```python
from build123d import *

# Parameters (mm, degrees)
SKETCH1_W           = 202.8
SKETCH1_H           = 130.8
SKETCH1_W_2         = 198
SKETCH1_H_2         = 126
BOSS_EXTRUDE1_DEPTH = 102
SKETCH3_W           = 198
SKETCH3_H           = 126
BOSS_EXTRUDE3_DEPTH = 2.4
FILLET1_R           = 5
FILLET4_R           = 10
FILLET2_R           = 6
FILLET3_R           = 0.4
CUT_EXTRUDE1_DEPTH  = 30


with BuildPart() as part:
    # Sketch1 → Boss-Extrude1 (new body)
    with BuildSketch(Plane(origin=(0, 0, 0), x_dir=(1, 0, 0), z_dir=(0, 1, 0))):
        with Locations((99, -63)):
            Rectangle(SKETCH1_W, SKETCH1_H)
        with Locations((99, -63)):
            Rectangle(SKETCH1_W_2, SKETCH1_H_2, mode=Mode.SUBTRACT)
    extrude(amount=BOSS_EXTRUDE1_DEPTH)

    # Sketch3 → Boss-Extrude3 (add)
    with BuildSketch(Plane(origin=(0, 0, 0), x_dir=(-1, 0, 0), z_dir=(0, -1, 0))):
        with Locations((-99, -63)):
            Rectangle(SKETCH3_W, SKETCH3_H)
    extrude(amount=-BOSS_EXTRUDE3_DEPTH)

    # Fillet1
    fillet1_edges = [part.edges().sort_by_distance(p)[0] for p in [
        (0, 2.4, 63),
        (99, 2.4, 126),
        (198, 2.4, 63),
        (99, 2.4, 0),
    ]]
    fillet(fillet1_edges, radius=FILLET1_R)

    # Fillet4
    # the kernel refuses this fillet: 10 mm, written as the material it adds along each edge
    with BuildSketch(Plane(origin=(10, 2.4, 10), x_dir=(-1, 0, 0), z_dir=(0, 0, 1))) as fillet4_piece_1:
        with BuildLine():
            CenterArc((5, -5), 5, 0, 90)
            Line((10, -5), (10, 0))
            Line((10, 0), (5, 0))
        make_face()
    revolve(axis=Axis((10, 2.4, 10), (0, -1, 0)), revolution_arc=90)
    with BuildSketch(Plane(origin=(10, 2.4, 116), x_dir=(0, 0, 1), z_dir=(1, 0, 0))) as fillet4_piece_2:
        with BuildLine():
            CenterArc((5, -5), 5, 0, 90)
            Line((10, -5), (10, 0))
            Line((10, 0), (5, 0))
        make_face()
    revolve(axis=Axis((10, 2.4, 116), (0, -1, 0)), revolution_arc=90)
    with BuildSketch(Plane(origin=(188, 2.4, 10), x_dir=(0, 0, -1), z_dir=(-1, 0, 0))) as fillet4_piece_3:
        with BuildLine():
            CenterArc((5, -5), 5, 0, 90)
            Line((10, -5), (10, 0))
            Line((10, 0), (5, 0))
        make_face()
    revolve(axis=Axis((188, 2.4, 10), (0, -1, 0)), revolution_arc=90)
    with BuildSketch(Plane(origin=(188, 2.4, 116), x_dir=(1, 0, 0), z_dir=(0, 0, -1))) as fillet4_piece_4:
        with BuildLine():
            CenterArc((5, -5), 5, 0, 90)
            Line((10, -5), (10, 0))
            Line((10, 0), (5, 0))
        make_face()
    revolve(axis=Axis((188, 2.4, 116), (0, -1, 0)), revolution_arc=90)
    with BuildSketch(Plane(origin=(0, 2.4, 0), x_dir=(1, 0, 0), z_dir=(0, 1, 0)), Plane(origin=(0, 2.4, 126), x_dir=(0, 0, -1), z_dir=(0, 1, 0))) as fillet4_piece_5:
        with BuildLine():
            CenterArc((FILLET4_R, -FILLET4_R), FILLET4_R, 90, 90)
            Line((0, -FILLET4_R), (0, 0))
            Line((0, 0), (FILLET4_R, 0))
        make_face()
    extrude(amount=99.6)
    with BuildSketch(Plane(origin=(198, 2.4, 126), x_dir=(0, 0, -1), z_dir=(0, 1, 0)), Plane(origin=(198, 2.4, 0), x_dir=(-1, 0, 0), z_dir=(0, 1, 0))) as fillet4_piece_6:
        with BuildLine():
            CenterArc((FILLET4_R, FILLET4_R), FILLET4_R, 180, 90)
            Line((0, FILLET4_R), (0, 0))
            Line((0, 0), (FILLET4_R, 0))
        make_face()
    extrude(amount=99.6)

    # Fillet2
    fillet2_edges = [part.edges().sort_by_distance(p)[0] for p in [
        (200.4, 51, -2.4),
        (200.4, 51, 128.4),
        (-2.4, 51, 128.4),
        (-2.4, 51, -2.4),
    ]]
    fillet(fillet2_edges, radius=FILLET2_R)

    # Fillet3
    fillet3_edges = [part.edges().sort_by_distance(p)[0] for p in [
        (99, 0, -2.4),
        (200.4, 0, 63),
        (-2.4, 0, 63),
        (198.642640687, 0, 126.642640687),
        (198.642640687, 0, -0.642640687),
        (-0.642640687, 0, -0.642640687),
        (-0.642640687, 0, 126.642640687),
        (99, 0, 128.4),
    ]]
    fillet(fillet3_edges, radius=FILLET3_R)

    # Sketch7 → Cut-Extrude1 (cut)
    with BuildSketch(Plane(origin=(0, 102, 0), x_dir=(1, 0, 0), z_dir=(0, 1, 0))):
        with BuildLine():
            Line((3.6, -127.2), (194.4, -127.2))
            ThreePointArc((194.4, -127.2), (197.79411255, -125.79411255), (199.2, -122.4))
            Line((199.2, -122.4), (199.2, -3.6))
            ThreePointArc((199.2, -3.6), (197.79411255, -0.20588745), (194.4, 1.2))
            Line((194.4, 1.2), (3.6, 1.2))
            ThreePointArc((3.6, 1.2), (0.20588745, -0.20588745), (-1.2, -3.6))
            Line((-1.2, -3.6), (-1.2, -122.4))
            ThreePointArc((-1.2, -122.4), (0.20588745, -125.79411255), (3.6, -127.2))
        make_face()
    extrude(amount=-CUT_EXTRUDE1_DEPTH, mode=Mode.SUBTRACT)


solid = part.part
```
The model under review builds one solid part; all positions refer to its coordinate system, in mm. A direction names the side the tool comes from. Round coordinates to 2 decimals unless told otherwise and drop trailing zeros. Write each loop counter-clockwise with the first axis right and the second up, starting at its lowest first coordinate (ties: lowest second). Pieces come first, ordered by that corner, then holes. Notation, with made-up numbers: (11, -22.5) - (63, -22.5) arc R12 ccw to (63, -9.5) - close; hole circle Ø9 at (41, -28.5). An arc over 180 degrees is marked (long way). Use one line per item in the form item = value.
Q1. For line 1 (Z direction, x = 13, y = 49); line 2 (X direction, y = 27, z = 37.5); line 3 (X direction, y = 95.5, z = 111), list the stretches that pass through material, from the lowest coordinate up. Write a range as [from, to].
Answer key:
line_1 = [-2.4, 0], [126, 128.4]
line_2 = [-2.4, 0], [198, 200.4]
line_3 = [-2.4, -1.2], [199.2, 200.4]
Q2. Tool access review of faces 4 (the flat face through (98, 87, 127.2)), 5 (the flat face through (98, 50, 128.4)): name each direction out of +Z, -Z, +X, -X, +Y, -Y from which nothing blocks a thin tool from reaching the whole face with its end or side.
Answer key:
face_4 = +Y
face_5 = +Z, +X, -X, +Y, -Y
Q3. Insertion check: pin 1 Ø4 at (x, z) = (33, 24) entering from +Y. The pin has a flat end and moves straight along its axis. Give the tip position at first contact, or say it passes through.
Answer key:
pin_1 = 2.4
Q4. Consider section B-B (z = 47). State the section outline as (x, y) points, and give its area (3 significant figures).
Answer key:
outline = (-2.4, 0.4) arc R0.4 ccw to (-2, 0) - (200, 0) arc R0.4 ccw to (200.4, 0.4) - (200.4, 102) - (199.2, 102) - (199.2, 72) - (198, 72) - (198, 7.4) arc R5 cw to (193, 2.4) - (5, 2.4) arc R5 cw to (0, 7.4) - (0, 72) - (-1.2, 72) - (-1.2, 102) - (-2.4, 102) - close
area = 903 mm2
Q5. Consider section C-C (x = 84). State the section outline as (y, z) points, and give its area (3 significant figures).
Answer key:
outline = (0, -2) arc R0.4 ccw to (0.4, -2.4) - (102, -2.4) - (102, -1.2) - (72, -1.2) - (72, 0) - (7.4, 0) arc R5 cw to (2.4, 5) - (2.4, 121) arc R5 cw to (7.4, 126) - (72, 126) - (72, 127.2) - (102, 127.2) - (102, 128.4) - (0.4, 128.4) arc R0.4 ccw to (0, 128) - close
area = 731 mm2
Q6. Draft analysis for pull direction Z (two halves, no side actions). For faces 1 (the flat face through (200.4, 50, 64)), 2 (the cylindrical face through (-0.689, 51.911, 126.596)), 3 (the cylindrical face through (97.75, 3.9, 124.57)), state which applies: +Z half, -Z half, draft (parallel to the pull), parting line (faces both ways), or undercut.
Answer key:
face_1 = draft
face_2 = +Z half
face_3 = undercut
Q7. Consider section D-D (y = 84). State the section outline as (x, z) points, and give its area (3 significant figures).
Answer key:
outline = (-2.4, 3.6) arc R6 ccw to (3.6, -2.4) - (194.4, -2.4) arc R6 ccw to (200.4, 3.6) - (200.4, 122.4) arc R6 ccw to (194.4, 128.4) - (3.6, 128.4) arc R6 ccw to (-2.4, 122.4) - close; hole (-1.2, 3.6) arc R4.8 ccw to (3.6, -1.2) - (194.4, -1.2) arc R4.8 ccw to (199.2, 3.6) - (199.2, 122.4) arc R4.8 ccw to (194.4, 127.2) - (3.6, 127.2) arc R4.8 ccw to (-1.2, 122.4) - close
area = 784 mm2
Q8. Consider section A-A (y = 69). State the section outline as (x, z) points, and give its area (3 significant figures).
Answer key:
outline = (-2.4, 3.6) arc R6 ccw to (3.6, -2.4) - (194.4, -2.4) arc R6 ccw to (200.4, 3.6) - (200.4, 122.4) arc R6 ccw to (194.4, 128.4) - (3.6, 128.4) arc R6 ccw to (-2.4, 122.4) - close; hole (0, 10) arc R10 ccw to (10, 0) - (188, 0) arc R10 ccw to (198, 10) - (198, 116) arc R10 ccw to (188, 126) - (10, 126) arc R10 ccw to (0, 116) - close
area = 1,630 mm2
